from build123d import *

# Parameters (mm, degrees)
SKETCH002_W  = 177
SKETCH002_H  = 16
SKETCH002_R  = 8
PAD002_DEPTH = 18
FILLET_R     = 5
SKETCH_W     = 18
SKETCH_H     = 70
POCKET_DEPTH = 145


with BuildPart() as part:
    # Sketch002 → Pad002 (new body)
    with BuildSketch(Plane.YZ.offset(132)):
        Polygon((-130, 10), (-130, 142), (130, 142), (130, 10), (88.5, 10), (88.5, 28), (-88.5, 28), (-88.5, 10), align=None)
        with Locations((0, 45)):
            Rectangle(SKETCH002_W, SKETCH002_H, mode=Mode.SUBTRACT)
        with Locations((-83.20224, 122.196114)):
            Circle(SKETCH002_R, mode=Mode.SUBTRACT)
        with Locations((-59.318291, 122.57251)):
            Circle(SKETCH002_R, mode=Mode.SUBTRACT)
        with Locations((60.411636, 121.713104)):
            Circle(SKETCH002_R, mode=Mode.SUBTRACT)
        with Locations((82.951927, 121.552109)):
            Circle(SKETCH002_R, mode=Mode.SUBTRACT)
    extrude(amount=PAD002_DEPTH)

    # Fillet
    fillet_edges = [part.edges().sort_by_distance(p)[0] for p in [
        (150, -130, 76),
        (150, 130, 76),
    ]]
    fillet(fillet_edges, radius=FILLET_R)

    # Sketch → Pocket (cut)
    with BuildSketch(Plane.YZ):
        with Locations((-97, 35)):
            Rectangle(SKETCH_W, SKETCH_H)
        with Locations((97, 35)):
            Rectangle(SKETCH_W, SKETCH_H)
    extrude(amount=POCKET_DEPTH, mode=Mode.SUBTRACT)


solid = part.part
The model under review builds one solid part; all positions refer to its coordinate system, in mm. A direction names the side the tool comes from. Coordinates: 2 decimals unless noted, no trailing zeros. Write each loop counter-clockwise with the first axis right and the second up, starting at its lowest first coordinate (ties: lowest second). Pieces come first, ordered by that corner, then holes. Notation, with made-up numbers: (-10, 45.5) -> (34, 45.5) arc R8 cw to (34, 51.5) -> close; hole circle Ø1 at (79, 13.25). An arc over 180 degrees is marked (long way). Answer in a Markdown table with one row per item.
1. We need section C-C, the plane y = -57. State the section outline as (x, z) points, and give its area (3 significant figures).
Answers below:
| item | result |
|---|---|
| outline | (132, 28) -> (150, 28) -> (150, 37) -> (132, 37) -> close; (132, 53) -> (150, 53) -> (150, 114.92) -> (132, 114.92) -> close; (132, 130.23) -> (150, 130.23) -> (150, 142) -> (132, 142) -> close |
| area | 1,490 mm^2 |
2. We need section B-B, the plane x = 136.75. State the section outline as (y, z) points, and give its area (3 significant figures).
Answers below:
| item | result |
|---|---|
| outline | (-130, 10) -> (-106, 10) -> (-106, 70) -> (-88, 70) -> (-88, 53) -> (88, 53) -> (88, 70) -> (106, 70) -> (106, 10) -> (130, 10) -> (130, 142) -> (-130, 142) -> close; (-88, 28) -> (88, 28) -> (88, 37) -> (-88, 37) -> close; hole circle Ø16 at (-83.2, 122.2); hole circle Ø16 at (-59.32, 122.57); hole circle Ø16 at (60.41, 121.71); hole circle Ø16 at (82.95, 121.55) |
| area | 25,400 mm^2 |
3. Draft analysis for pull direction Y (two halves, no side actions). For faces 1 (the flat face through (150, 2, 77)), 2 (the flat face through (141, -1, 37)), 3 (the flat face through (138, -130, 75)), state which applies: +Y half, -Y half, draft (parallel to the pull), parting line (faces both ways), or undercut.
Answers below:
| item | result |
|---|---|
| face 1 | draft |
| face 2 | undercut |
| face 3 | -Y half |
4. Clearance check with flat-ended pins moving along their axes: pin 1 Ø1.5 at (x, z) = (148.5, 16.5) entering from -Y; pin 2 Ø1.5 at (x, z) = (148.5, 16) entering from +Y; pin 3 Ø6.5 at (x, y) = (140.5, -100.5) entering from -Z. State where each tip first meets the part, or that it passes through.
Answers below:
| item | result |
|---|---|
| pin 1 | stops at y = -129.18 |
| pin 2 | stops at y = 129.18 |
| pin 3 | stops at z = 70 |
5. We need section A-A, the plane y = 26. State the section outline as (x, z) points.
Answers below:
| item | result |
|---|---|
| outline | (132, 28) -> (150, 28) -> (150, 37) -> (132, 37) -> close; (132, 53) -> (150, 53) -> (150, 142) -> (132, 142) -> close |
6. Wall thickness on probe 1 along Y at (x, z) = (137, 66); probe 2 along Y at (x, z) = (143.75, 38.5); probe 3 along Z at (x, y) = (142.75, 84.5): over which ranges is each line inside the solid? List them lowest first. Write a range as [from, to].
Answers below:
| item | result |
|---|---|
| probe 1 | y = [-130, -106], [-88, 88], [106, 130] |
| probe 2 | y = [-130, -106], [106, 130] |
| probe 3 | z = [28, 37], [53, 113.7], [129.4, 142] |
7. We need section D-D, the plane y = 65. State the section outline as (x, z) points, and give its area (3 significant figures).
Answers below:
| item | result |
|---|---|
| outline | (132, 28) -> (150, 28) -> (150, 37) -> (132, 37) -> close; (132, 53) -> (150, 53) -> (150, 115.16) -> (132, 115.16) -> close; (132, 128.27) -> (150, 128.27) -> (150, 142) -> (132, 142) -> close |
| area | 1,530 mm^2 |
8. For faces 4 (the flat face through (145, 97, 40)), 5 (the cylindrical face through (148, -129, 77)), 6 (the flat face through (141, -1, 53)), 7 (the cylindrical face through (148, 129, 75)), 8 (the flat face through (147, -88.5, 19)), list the 3-axis set-ups (+Z, -Z, +X, -X, +Y, -Y) from which the entire face can be reached by the end or side of a thin tool; tool diameter is ignored.
Answers below:
| item | result |
|---|---|
| face 4 | -Z, -X |
| face 5 | +Z, -Z, +X, -Y |
| face 6 | +X, -X |
| face 7 | +Z, -Z, +X, +Y |
| face 8 | -Z, +X, -X |
